Geometry: final body of the model. Coordinates: model frame, mm. Coordinates: 2 decimals unless noted, no trailing zeros. Order: outer loops, then holes, each group sorted by start corner. A loop starts at its lowest first (then second) coordinate and runs counter-clockwise, first axis right, second up. Notation, with made-up numbers: (-21.5, 18) - (9.5, 18) arc R28 ccw to (9.5, 49) - close; hole circle Ø8 at (-7, 87). An arc over 180 degrees is marked (long way). Use a Markdown table: item, result. Add a question column.
```python
from build123d import *

# Parameters (mm, degrees)
SKETCH1_R           = 0.65
BOSS_EXTRUDE1_DEPTH = 0.8
BOSS_EXTRUDE2_DEPTH = 1.4
BOSS_EXTRUDE3_DEPTH = 0.8
SKETCH1_3_R         = 0.65
BOSS_EXTRUDE4_DEPTH = 3.9


with BuildPart() as part:
    # Sketch1 → Boss-Extrude1 (new body)
    # profile 1 of 5: a face of its own
    with BuildSketch(Plane(origin=(0, 0, 0), x_dir=(1, 0, 0), z_dir=(0, 1, 0))):
        with BuildLine():
            ThreePointArc((-165.584512428, 53.801669479), (-174.105859737, 0), (-165.584512428, -53.801669479))
            Line((-165.584512428, -53.801669479), (-167.962153719, -54.574211965))
            ThreePointArc((-167.962153719, -54.574211965), (-176.605859737, 0), (-167.962153719, 54.574211965))
            Line((-167.962153719, 54.574211965), (-165.584512428, 53.801669479))
        make_face()
        with Locations((-172.538, -31.31)):
            Circle(SKETCH1_R, mode=Mode.SUBTRACT)
    # profile 2 of 5: a face of its own
    with BuildSketch(Plane(origin=(0, 0, 0), x_dir=(1, 0, 0), z_dir=(0, 1, 0))):
        with Locations((-172.538, -31.31)):
            Circle(SKETCH1_R)
    # profile 3 of 5: a face of its own
    with BuildSketch(Plane(origin=(0, 0, 0), x_dir=(1, 0, 0), z_dir=(0, 1, 0))):
        with Locations((-167.932, -50.621)):
            Circle(SKETCH1_R)
    # profile 4 of 5: a face of its own
    with BuildSketch(Plane(origin=(0, 0, 0), x_dir=(1, 0, 0), z_dir=(0, 1, 0))):
        with Locations((-172.538, 31.31)):
            Circle(SKETCH1_R)
    # profile 5 of 5: a face of its own
    with BuildSketch(Plane(origin=(0, 0, 0), x_dir=(1, 0, 0), z_dir=(0, 1, 0))):
        with Locations((-167.932, 50.621)):
            Circle(SKETCH1_R)
    extrude(amount=BOSS_EXTRUDE1_DEPTH)

    # Sketch2 → Boss-Extrude2 (add)
    with BuildSketch(Plane(origin=(0, 0.8, 0), x_dir=(1, 0, 0), z_dir=(0, 1, 0))):
        with BuildLine():
            Line((-165.869829383, 53.894374577), (-167.676836764, 54.481506867))
            ThreePointArc((-167.676836764, 54.481506867), (-176.305859737, 0), (-167.676836764, -54.481506867))
            Line((-167.676836764, -54.481506867), (-165.869829383, -53.894374577))
            ThreePointArc((-165.869829383, -53.894374577), (-174.405859737, 0), (-165.869829383, 53.894374577))
        make_face()
    extrude(amount=BOSS_EXTRUDE2_DEPTH)

    # Sketch3 → Boss-Extrude3 (add)
    with BuildSketch(Plane(origin=(0, 2.2, 0), x_dir=(1, 0, 0), z_dir=(0, 1, 0))):
        with BuildLine():
            Line((-167.962153719, -54.574211965), (-165.584512428, -53.801669479))
            ThreePointArc((-165.584512428, -53.801669479), (-174.105859737, 0), (-165.584512428, 53.801669479))
            Line((-165.584512428, 53.801669479), (-167.962153719, 54.574211965))
            ThreePointArc((-167.962153719, 54.574211965), (-176.605859737, 0), (-167.962153719, -54.574211965))
        make_face()
    extrude(amount=BOSS_EXTRUDE3_DEPTH)

    # Sketch1_3 → Boss-Extrude4 (add)
    with BuildSketch(Plane(origin=(0, 0, 0), x_dir=(1, 0, 0), z_dir=(0, 1, 0))):
        with Locations(Location((-172.538, -31.31, 0), (0, 0, 270))):
            Circle(SKETCH1_3_R)
        with Locations(Location((-167.932, 50.621, 0), (0, 0, 270))):
            Circle(SKETCH1_3_R)
        with Locations(Location((-167.932, -50.621, 0), (0, 0, 270))):
            Circle(SKETCH1_3_R)
        with Locations(Location((-172.538, 31.31, 0), (0, 0, 270))):
            Circle(SKETCH1_3_R)
    extrude(amount=BOSS_EXTRUDE4_DEPTH)


solid = part.part
```
1) Draft query along Y for faces 1 (the cylindrical face through (-176.604, 0.394, 0.777)), 2 (the cylindrical face through (-174.404, 1.49, 0.767)), 3 (the cylindrical face through (-176.304, 1.49, -0.775)), 4 (the flat face through (-174.4, 3, -0.3)). Return one class per face: released by +Y, released by -Y, zero draft, split by the parting line, or undercut.
2) Section query C-C (y = 1.4). Return the cut outline in (x, z).
3) Section query D-D (z = 13). Return the cut outline in (x, y).
4) First-contact query: pin 1 (1 mm diameter, centred on y = 2, z = -8.5, fed in from +X). Flat tip, straight axial feed; report the tip coordinate or a pass-through.
5) Section query B-B (z = -9). Return the cut outline in (x, y), and give its area (3 significant figures).
6) Section query A-A (x = -170). Return the cut outline in (y, z).
7) Line query: line 1 (Y direction, x = -168, z = 48); line 2 (X direction, y = 1.05, z = 38.5); line 3 (X direction, y = 2.25, z = -27.5). Output: solid intervals per line, ascending. Write a range as from..to.
From the geometry:
| question | item | result |
|---|---|---|
| 1 | face 1 | zero draft |
| 1 | face 2 | undercut |
| 1 | face 3 | undercut |
| 1 | face 4 | released by +Y |
| 2 | outline | (-167.68, -54.48) - (-165.87, -53.89) arc R174.41 cw to (-165.87, 53.89) - (-167.68, 54.48) arc R176.31 ccw to start |
| 3 | outline | (-176.13, 0) - (-173.62, 0) - (-173.62, 0.8) - (-173.92, 0.8) - (-173.92, 2.2) - (-173.62, 2.2) - (-173.62, 3) - (-176.13, 3) - (-176.13, 2.2) - (-175.83, 2.2) - (-175.83, 0.8) - (-176.13, 0.8) - close |
| 4 | pin 1 | stops at x = -173.88 |
| 5 | outline | (-176.38, 0) - (-173.87, 0) - (-173.87, 0.8) - (-174.17, 0.8) - (-174.17, 2.2) - (-173.87, 2.2) - (-173.87, 3) - (-176.38, 3) - (-176.38, 2.2) - (-176.08, 2.2) - (-176.08, 0.8) - (-176.38, 0.8) - close |
| 5 | area | 6.67 mm^2 |
| 6 | outline | (0, -47.85) - (0.8, -47.85) - (0.8, -46.73) - (2.2, -46.73) - (2.2, -47.85) - (3, -47.85) - (3, -37.59) - (2.2, -37.59) - (2.2, -38.95) - (0.8, -38.95) - (0.8, -37.59) - (0, -37.59) - close; (0, 37.59) - (0.8, 37.59) - (0.8, 38.95) - (2.2, 38.95) - (2.2, 37.59) - (3, 37.59) - (3, 47.85) - (2.2, 47.85) - (2.2, 46.73) - (0.8, 46.73) - (0.8, 47.85) - (0, 47.85) - close |
| 7 | line 1 | y = 0..3 |
| 7 | line 2 | x = -172.05..-170.1 |
| 7 | line 3 | x = -174.45..-171.92 |
